from build123d import *

# Parameters (mm, degrees)
F2_DEPTH  = 41
F1_W      = 1.7
F1_H      = 47.8
F1_W_2    = 77.3
F3_DEPTH  = 3
F1_W_3    = 2.5
F1_H_2    = 1.7
F4_DEPTH  = 1.5
F5_W      = 14.41
F5_H      = 12
F5_W_2    = 10.4
F6_DEPTH  = 3
F7_W      = 1.4
F7_H      = 2
F8_DEPTH  = 81
F9_W      = 1.7
F9_H      = 2.5
F10_DEPTH = 83
F11_W     = 47.8
F11_H     = 2.5
F12_DEPTH = 1.5


with BuildPart() as f2:
    # F1 (on Top) → F2 (new body)
    with BuildSketch(Plane.XY):
        Polygon((-43, 27.4), (-43, 23.9), (-41.3, 23.9), (-41.3, 25.6), (-38.8, 25.6), (-38.8, 23.9), (38.5, 23.9), (38.5, -23.9), (-38.8, -23.9), (-38.8, -25.6), (-41.3, -25.6), (-41.3, -23.9), (-43, -23.9), (-43, -27.4), (40.8, -27.4), (40.8, 27.4), align=None)
    extrude(amount=F2_DEPTH)

    # F1 (on Top) → F3 (join)
    with BuildSketch(Plane.XY):
        with Locations((-42.15, 0)):
            Rectangle(F1_W, F1_H)
        with Locations((-0.15, 0)):
            Rectangle(F1_W_2, F1_H)
    extrude(amount=F3_DEPTH)

    # F1 (on Top) → F4 (join)
    with BuildSketch(Plane.XY):
        with Locations((-40.05, -24.75)):
            Rectangle(F1_W_3, F1_H_2)
        with Locations((-40.05, 0)):
            Rectangle(F1_W_3, F1_H)
        with Locations((-40.05, 24.75)):
            Rectangle(F1_W_3, F1_H_2)
    extrude(amount=F4_DEPTH)

    # F5 (on face) → F6 (cut)
    with BuildSketch(Plane.YZ.offset(40.8)):
        with Locations((-7.065, 9)):
            Rectangle(F5_W, F5_H)
        with Locations((11, 9)):
            Rectangle(F5_W_2, F5_H)
    extrude(amount=-F6_DEPTH, mode=Mode.SUBTRACT)

    # F7 (on face) → F8 (cut)
    with BuildSketch(Plane(origin=(-43, 0, 0), x_dir=(0, -1, 0), z_dir=(-1, 0, 0))):
        with Locations((-24.6, 15.5)):
            Rectangle(F7_W, F7_H)
        with Locations((-24.6, 22.45)):
            Rectangle(F7_W, F7_H)
        with Locations((24.6, 15.5)):
            Rectangle(F7_W, F7_H)
        with Locations((24.6, 22.45)):
            Rectangle(F7_W, F7_H)
    extrude(amount=-F8_DEPTH, mode=Mode.SUBTRACT)

    # F9 (on face) → F10 (cut)
    with BuildSketch(Plane(origin=(-43, 0, 0), x_dir=(0, -1, 0), z_dir=(-1, 0, 0))):
        with Locations((-24.75, 38.05)):
            Rectangle(F9_W, F9_H)
        with Locations((24.75, 38.05)):
            Rectangle(F9_W, F9_H)
    extrude(amount=-F10_DEPTH, mode=Mode.SUBTRACT)

    # F11 (on face) → F12 (cut)
    with BuildSketch(Plane(origin=(38.5, 0, 0), x_dir=(0, -1, 0), z_dir=(-1, 0, 0))):
        with Locations((0, 38.05)):
            Rectangle(F11_W, F11_H)
    extrude(amount=-F12_DEPTH, mode=Mode.SUBTRACT)


solid = f2.part
Work out the finished part from the listing and answer in its coordinate system (mm). A direction names the side the tool comes from. Coordinates: 2 decimals unless noted, no trailing zeros. Loops run counter-clockwise (first coordinate to the right, second up) from the corner with the lowest first, then second, coordinate; pieces in that order, holes last. Notation, with made-up numbers: (56, 58) -> (88, 58) arc R35 cw to (88, 96) -> close; hole circle Ø1 at (1, 64.25). An arc over 180 degrees is marked (long way). Write each question's results on one line, items separated by ' | '. Start each with the question number.
1) For faces 1 (the flat face through (-38.8, -25, 40)), 2 (the flat face through (-42, 0, 3)), 3 (the flat face through (40, 11, 15)), 4 (the flat face through (0, 25, 36.8)), determine the directions among +Z, -Z, +X, -X, +Y, -Y from which every point of the face is accessible in a straight line to the end or side of a thin tool.
2) Find section B-B on z = 5.5. Determine the outline of the cut face in (x, y), then the cut area to 3 significant figures.
3) The mould has two halves that part along X. Classify faces 5 (the flat face through (-41.3, 0, 2)), 6 (the flat face through (-43, -2, 2)), 7 (the flat face through (-42, 23.9, 9)): pulls with the +X half, pulls with the -X half, needs draft (parallel to the pull), parting line crosses it, or undercut.
4) Flat-ended cylindrical pins translate along their axes: P1, Ø3, axis at x = 9, y = 7.5, coming from the +Z side; P2, Ø1, axis at y = -8, z = 4.5, coming from the +X side; P3, Ø17, axis at y = 7, z = 16, coming from the -X side; P4, Ø2, axis at x = -33, y = -13, coming from the -Z side. Find the tip coordinate at first contact, or state that the pin passes through.
5) Find section A-A on y = -5.5. Determine the outline of the cut face in (x, z), then the cut area to 3 significant figures.
6) Find section D-D on y = -23. Determine the outline of the cut face in (x, z).
7) Consider line 1 along Y through (x, z) = (3, 12); line 2 along X through (y, z) = (-4, 28); line 3 along Z through (x, y) = (-5, -12.5). Determine where each line is inside the solid, lowest interval first.
Response values:
1) face 1: +Z | face 2: +Z, -X | face 3: +X, -X | face 4: -X
2) outline: (-43, -27.4) -> (40.8, -27.4) -> (40.8, -14.27) -> (38.5, -14.27) -> (38.5, -23.9) -> (-38.8, -23.9) -> (-38.8, -25.6) -> (-41.3, -25.6) -> (-41.3, -23.9) -> (-43, -23.9) -> close; (-43, 23.9) -> (-41.3, 23.9) -> (-41.3, 25.6) -> (-38.8, 25.6) -> (-38.8, 23.9) -> (38.5, 23.9) -> (38.5, 16.2) -> (40.8, 16.2) -> (40.8, 27.4) -> (-43, 27.4) -> close; (38.5, 0.14) -> (40.8, 0.14) -> (40.8, 5.8) -> (38.5, 5.8) -> close | area: 631 mm^2
3) face 5: undercut | face 6: pulls with the -X half | face 7: needs draft
4) P1: stops at z = 3 | P2: passes through | P3: stops at x = 38.5 | P4: stops at z = 0
5) outline: (-43, 0) -> (40.8, 0) -> (40.8, 3) -> (-38.8, 3) -> (-38.8, 1.5) -> (-41.3, 1.5) -> (-41.3, 3) -> (-43, 3) -> close; (38.5, 15) -> (40.8, 15) -> (40.8, 41) -> (38.5, 41) -> (38.5, 39.3) -> (40, 39.3) -> (40, 36.8) -> (38.5, 36.8) -> close | area: 304 mm^2
6) outline: (-43, 0) -> (40.8, 0) -> (40.8, 41) -> (38.5, 41) -> (38.5, 39.3) -> (40, 39.3) -> (40, 36.8) -> (38.5, 36.8) -> (38.5, 3) -> (-38.8, 3) -> (-38.8, 1.5) -> (-41.3, 1.5) -> (-41.3, 3) -> (-43, 3) -> close
7) line 1: y = -27.4 to -23.9, 23.9 to 27.4 | line 2: x = 38.5 to 40.8 | line 3: z = 0 to 3
